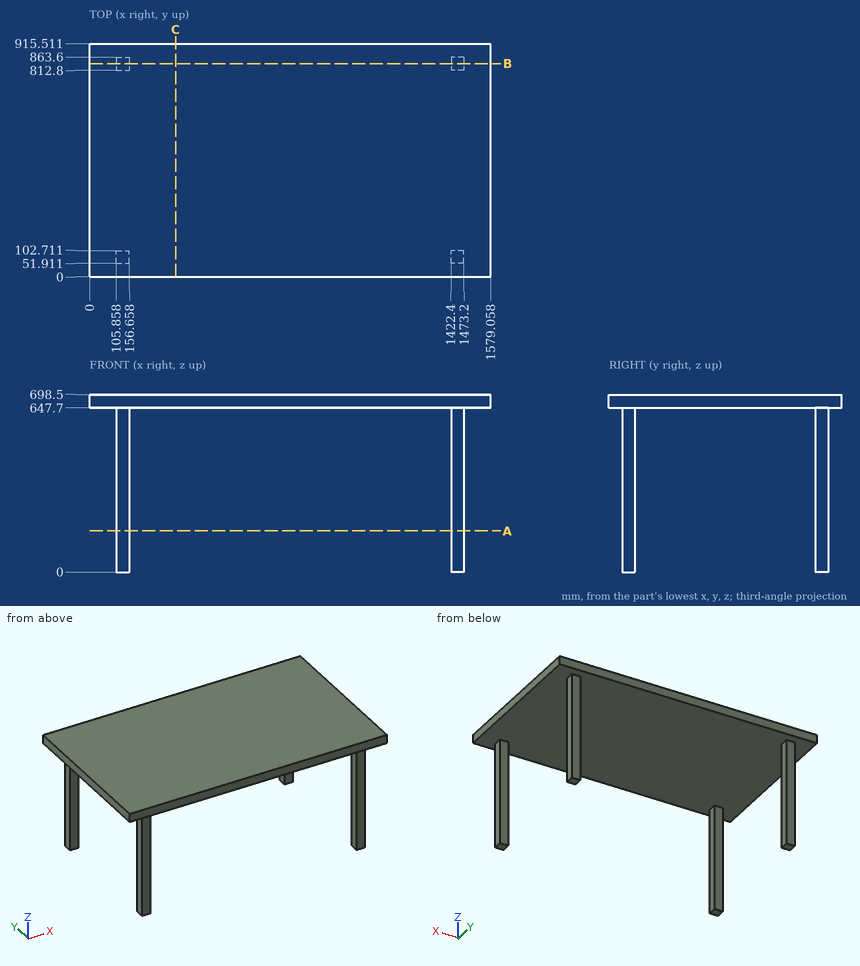
Answer from the drawing. Dimensions are ordinates in mm from the lowest x, y and z of the part. Round coordinates to 2 decimals unless told otherwise and drop trailing zeros. Write each loop counter-clockwise with the first axis right and the second up, starting at its lowest first coordinate (ties: lowest second). Pieces come first, ordered by that corner, then holes. Notation, with made-up numbers: M -26.5,77 L 31.5,77 A32 cw 31.5,107 Z; hole C -16,30 d2. An arc over 180 degrees is marked long. Write each question's results on one line, items separated by ' | '. Start each with the question number.
Item 1: Find section B-B on y = 838.5. Write down the section's boundary in (x, z).
Item 2: Given pin 1 Ø15 at (y, z) = (69.5, 325) entering from -X; pin 2 Ø15 at (x, z) = (144, 319) entering from -Y, each flat-ended and moving along its own axis, determine where each tip first touches the part or whether it passes through.
Item 3: Find section A-A on z = 162.5. Write down the section's boundary in (x, y), and give its area (3 significant figures).
Item 4: Find section C-C on x = 339. Write down the section's boundary in (y, z).
Item 5: Straight lines are drawn through the part: probe 1 along X at (y, z) = (817, 448); probe 2 along Z at (x, y) = (672, 254). For each, find the intervals that lie inside material, in ascending order.
Answer block:
1) outline: M 0,647.7 L 105.86,647.7 L 105.86,0 L 156.66,0 L 156.66,647.7 L 1422.4,647.7 L 1422.4,0 L 1473.2,0 L 1473.2,647.7 L 1579.06,647.7 L 1579.06,698.5 L 0,698.5 Z
2) pin 1: stops at x = 105.86 | pin 2: stops at y = 51.91
3) outline: M 105.86,51.91 L 156.66,51.91 L 156.66,102.71 L 105.86,102.71 Z; M 105.86,812.8 L 156.66,812.8 L 156.66,863.6 L 105.86,863.6 Z; M 1422.4,51.91 L 1473.2,51.91 L 1473.2,102.71 L 1422.4,102.71 Z; M 1422.4,812.8 L 1473.2,812.8 L 1473.2,863.6 L 1422.4,863.6 Z | area: 10,300 mm²
4) outline: M 0,647.7 L 915.51,647.7 L 915.51,698.5 L 0,698.5 Z
5) probe 1: x = 105.86 to 156.66, 1422.4 to 1473.2 | probe 2: z = 647.7 to 698.5
